```python
from build123d import *

# Parameters (mm, degrees)
BOSS_EXTRUDE1_DEPTH      = 203.2
BOSS_EXTRUDE1_DEPTH_BACK = 203.2
SKETCH1_R                = 4.953
BOSS_EXTRUDE2_DEPTH      = 177.8
BOSS_EXTRUDE2_DEPTH_BACK = 177.8


with BuildPart() as part:
    # Sketch1 → Boss-Extrude1 (new, two sides: drawn at the far end of the back side and taken through both)
    with BuildSketch(Plane.XY.offset(-BOSS_EXTRUDE1_DEPTH_BACK)):
        Circle(SKETCH1_R)
    extrude(amount=BOSS_EXTRUDE1_DEPTH + BOSS_EXTRUDE1_DEPTH_BACK)

    # Sketch2 → Boss-Extrude2 (add, two sides: drawn at the far end of the back side and taken through both)
    with BuildSketch(Plane.XY.offset(-BOSS_EXTRUDE2_DEPTH_BACK)):
        Polygon((5.719231767, 0), (2.859615883, 4.953), (-2.859615883, 4.953), (-5.719231767, 0), (-2.859615883, -4.953), (2.859615883, -4.953), align=None)
    extrude(amount=BOSS_EXTRUDE2_DEPTH + BOSS_EXTRUDE2_DEPTH_BACK)


solid = part.part
```
Geometry check sheet. Reference: the model listing, model coordinates, mm. A direction names the side the tool comes from. Give positions to 0.01 mm unless a question says otherwise; leave off trailing zeros. Write each loop counter-clockwise with the first axis right and the second up, starting at its lowest first coordinate (ties: lowest second). Pieces come first, ordered by that corner, then holes. Notation, with made-up numbers: (50, 16) -> (68, 16) arc R27 ccw to (68, 53) -> close; hole circle Ø7 at (-33, -35). An arc over 180 degrees is marked (long way). One line per question, with ' | ' between items.
Item 1: Access from +Z, -Z, +X, -X, +Y, -Y to the whole of each face (thin tool, end or side, straight path). Record for faces 1 (the cylindrical face through (-0.64, 4.91, 190.32)), 2 (the cylindrical face through (-0.64, 4.91, -190.68)), 3 (the flat face through (0, 0, -203.2)).
Determined:
face 1: +Z | face 2: -Z | face 3: -Z, +X, -X, +Y, -Y
Item 2: Sectioned sample at A-A, the plane z = 159. Record the boundary of the cut face in (x, y), plus the area to 3 significant figures.
Determined:
outline: (-5.72, 0) -> (-2.86, -4.95) -> (2.86, -4.95) -> (5.72, 0) -> (2.86, 4.95) -> (-2.86, 4.95) -> close | area: 85.0 mm^2
Item 3: Scan lines: line 1 along X through (y, z) = (2.5, 129); line 2 along Y through (x, z) = (4.5, -126.5); line 3 along X through (y, z) = (3, -109). Record each from-to range of solid material in increasing order.
Determined:
line 1: -4.28 to 4.28 | line 2: -2.11 to 2.11 | line 3: -3.99 to 3.99
Item 4: Depth check by flat-ended pin: pin 1 (2.5 mm diameter, centred on x = -3, y = -4, fed in from -Z). Enter the tip coordinate at first touch or a pass-through.
Determined:
pin 1: z = -203.2
